Check sheet for the modelled part. Datum: model origin and axes. Units: mm. Give positions to 0.01 mm unless a question says otherwise; leave off trailing zeros. Order: outer loops, then holes, each group sorted by start corner. A loop starts at its lowest first (then second) coordinate and runs counter-clockwise, first axis right, second up.
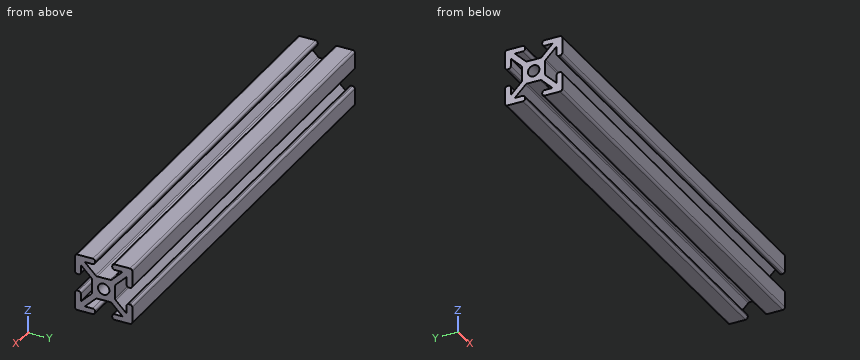
from build123d import *

# Parameters (mm, degrees)
SKETCH1_R           = 2
PROFILE_4X4_1_DEPTH = 150


with BuildPart() as part:
    # Sketch1 → Profile 4X4(1) (new body)
    with BuildSketch(Plane.YZ.offset(-67.810457516)):
        with BuildLine():
            Line((-3, 9.2), (-3, 8.8))
            ThreePointArc((-3, 8.8), (-3.234314575, 8.234314575), (-3.8, 8))
            Line((-3.8, 8), (-6.585786438, 8))
            Line((-6.585786438, 8), (-2.820101013, 4.234314575))
            ThreePointArc((-2.820101013, 4.234314575), (-2.560562334, 4.060896374), (-2.254415588, 4))
            Line((-2.254415588, 4), (2.254415588, 4))
            ThreePointArc((2.254415588, 4), (2.560562334, 4.060896374), (2.820101013, 4.234314575))
            Line((2.820101013, 4.234314575), (6.585786438, 8))
            Line((6.585786438, 8), (3.8, 8))
            ThreePointArc((3.8, 8), (3.234314575, 8.234314575), (3, 8.8))
            Line((3, 8.8), (3, 9.2))
            ThreePointArc((3, 9.2), (3.234314575, 9.765685425), (3.8, 10))
            Line((3.8, 10), (9.2, 10))
            ThreePointArc((9.2, 10), (9.765685425, 9.765685425), (10, 9.2))
            Line((10, 9.2), (10, 3.8))
            ThreePointArc((10, 3.8), (9.765685425, 3.234314575), (9.2, 3))
            Line((9.2, 3), (8.8, 3))
            ThreePointArc((8.8, 3), (8.234314575, 3.234314575), (8, 3.8))
            Line((8, 3.8), (8, 6.585786438))
            Line((8, 6.585786438), (4.234314575, 2.820101013))
            ThreePointArc((4.234314575, 2.820101013), (4.060896374, 2.560562334), (4, 2.254415588))
            Line((4, 2.254415588), (4, -2.254415588))
            ThreePointArc((4, -2.254415588), (4.060896374, -2.560562334), (4.234314575, -2.820101013))
            Line((4.234314575, -2.820101013), (8, -6.585786438))
            Line((8, -6.585786438), (8, -3.8))
            ThreePointArc((8, -3.8), (8.234314575, -3.234314575), (8.8, -3))
            Line((8.8, -3), (9.2, -3))
            ThreePointArc((9.2, -3), (9.765685425, -3.234314575), (10, -3.8))
            Line((10, -3.8), (10, -9.2))
            ThreePointArc((10, -9.2), (9.765685425, -9.765685425), (9.2, -10))
            Line((9.2, -10), (3.8, -10))
            ThreePointArc((3.8, -10), (3.234314575, -9.765685425), (3, -9.2))
            Line((3, -9.2), (3, -8.8))
            ThreePointArc((3, -8.8), (3.234314575, -8.234314575), (3.8, -8))
            Line((3.8, -8), (6.585786438, -8))
            Line((6.585786438, -8), (2.820101013, -4.234314575))
            ThreePointArc((2.820101013, -4.234314575), (2.560562334, -4.060896374), (2.254415588, -4))
            Line((2.254415588, -4), (-2.254415588, -4))
            ThreePointArc((-2.254415588, -4), (-2.560562334, -4.060896374), (-2.820101013, -4.234314575))
            Line((-2.820101013, -4.234314575), (-6.585786438, -8))
            Line((-6.585786438, -8), (-3.8, -8))
            ThreePointArc((-3.8, -8), (-3.234314575, -8.234314575), (-3, -8.8))
            Line((-3, -8.8), (-3, -9.2))
            ThreePointArc((-3, -9.2), (-3.234314575, -9.765685425), (-3.8, -10))
            Line((-3.8, -10), (-9.2, -10))
            ThreePointArc((-9.2, -10), (-9.765685425, -9.765685425), (-10, -9.2))
            Line((-10, -9.2), (-10, -3.8))
            ThreePointArc((-10, -3.8), (-9.765685425, -3.234314575), (-9.2, -3))
            Line((-9.2, -3), (-8.8, -3))
            ThreePointArc((-8.8, -3), (-8.234314575, -3.234314575), (-8, -3.8))
            Line((-8, -3.8), (-8, -6.585786438))
            Line((-8, -6.585786438), (-4.234314575, -2.820101013))
            ThreePointArc((-4.234314575, -2.820101013), (-4.060896374, -2.560562334), (-4, -2.254415588))
            Line((-4, -2.254415588), (-4, 2.254415588))
            ThreePointArc((-4, 2.254415588), (-4.060896374, 2.560562334), (-4.234314575, 2.820101013))
            Line((-4.234314575, 2.820101013), (-8, 6.585786438))
            Line((-8, 6.585786438), (-8, 3.8))
            ThreePointArc((-8, 3.8), (-8.234314575, 3.234314575), (-8.8, 3))
            Line((-8.8, 3), (-9.2, 3))
            ThreePointArc((-9.2, 3), (-9.765685425, 3.234314575), (-10, 3.8))
            Line((-10, 3.8), (-10, 9.2))
            ThreePointArc((-10, 9.2), (-9.765685425, 9.765685425), (-9.2, 10))
            Line((-9.2, 10), (-3.8, 10))
            ThreePointArc((-3.8, 10), (-3.234314575, 9.765685425), (-3, 9.2))
        make_face()
        Circle(SKETCH1_R, mode=Mode.SUBTRACT)
    extrude(amount=PROFILE_4X4_1_DEPTH)


solid = part.part
1) Section check A-A, the plane y = 0. Record the cut outline in (x, z).
Recorded:
outline: (-67.81, -4) - (82.19, -4) - (82.19, -2) - (-67.81, -2) - close; (-67.81, 2) - (82.19, 2) - (82.19, 4) - (-67.81, 4) - close
2) Depth check by flat-ended pin: pin 1 Ø4 at (x, y) = (16.5, -1.5) entering from -Z; pin 2 Ø1.4 at (x, z) = (28, 1) entering from +Y; pin 3 Ø1.4 at (x, z) = (33.5, 0.5) entering from -Y. Enter the tip coordinate at first touch or a pass-through.
Recorded:
pin 1: stops at z = -9.94
pin 2: stops at y = 4
pin 3: stops at y = -4
3) Material ranges on L1, parallel to Z at x = 43.5, y = 0; L2, parallel to Y at x = -56, z = 6; L3, parallel to Y at x = 42.5, z = 1.25, recorded low to high.
Recorded:
L1: z = -4 to -2, 2 to 4
L2: y = -10 to -8, -7.41 to -4.59, 4.59 to 7.41, 8 to 10
L3: y = -4 to -1.56, 1.56 to 4
